Design review of the part built by this model. Coordinates are the model's own, in mm. A direction names the side the tool comes from. Round coordinates to 2 decimals unless told otherwise and drop trailing zeros. Loops run counter-clockwise (first coordinate to the right, second up) from the corner with the lowest first, then second, coordinate; pieces in that order, holes last. Notation, with made-up numbers: (36.25, 66) -> (42.25, 66) arc R20 ccw to (42.25, 92) -> close; hole circle Ø7 at (25, -31). An arc over 180 degrees is marked (long way). Answer as CSV lines item,"result". Start each with the question number.
```python
from build123d import *

# Parameters (mm, degrees)
LOFT1_DEPTH = 254
LOFT1_DRAFT = -8.0697267
SHELL1_T    = -19.05


# Read off the part's stored shape, not the designer's step: Loft1
with BuildPart() as part:
    # Loft1 outline → Loft1 (with draft: the straight prism first)
    with BuildSketch(Plane(origin=(0, -254, 0), x_dir=(1, 0, 0), z_dir=(0, 1, 0))):
        Polygon((45.71024071, -79.172459336), (70.032151779, -58.763952728), (85.907151779, -31.267646158), (91.42048142, 0), (85.907151779, 31.267646158), (70.032151779, 58.763952728), (45.71024071, 79.172459336), (15.875, 90.031598886), (-15.875, 90.031598886), (-45.71024071, 79.172459336), (-70.032151779, 58.763952728), (-85.907151779, 31.267646158), (-91.42048142, 0), (-85.907151779, -31.267646158), (-70.032151779, -58.763952728), (-45.71024071, -79.172459336), (-15.875, -90.031598886), (15.875, -90.031598886), align=None)
    extrude(amount=LOFT1_DEPTH)
    # Loft1: the draft: its side faces are tilted about the plane it starts from
    loft1_sides = [part.faces().sort_by_distance(p)[0] for p in [
        (57.871196245, -127, 68.968206032),
        (77.969651779, -127, 45.015799443),
        (88.6638166, -127, 15.633823079),
        (88.663816599, -127, -15.633823079),
        (77.969651779, -127, -45.015799443),
        (57.871196244, -127, -68.968206032),
        (30.792620355, -127, -84.602029111),
        (0, -127, -90.031598886),
        (-30.792620355, -127, -84.602029111),
        (-57.871196245, -127, -68.968206032),
        (-77.969651779, -127, -45.015799443),
        (-88.6638166, -127, -15.633823079),
        (-88.663816599, -127, 15.633823079),
        (-77.969651779, -127, 45.015799443),
        (-57.871196244, -127, 68.968206032),
        (-30.792620355, -127, 84.602029111),
        (0, -127, 90.031598886),
        (30.792620355, -127, 84.602029111),
    ]]
    draft(loft1_sides, Plane(origin=(0, -254, 0), x_dir=(1, 0, 0), z_dir=(0, 1, 0)), LOFT1_DRAFT)

    # Shell1
    shell1_openings = [part.faces().sort_by_distance(p)[0] for p in [
        (0, 0, 0),
        (0, -254, 0),
    ]]
    offset(amount=SHELL1_T, openings=shell1_openings, kind=Kind.INTERSECTION)


solid = part.part
```
Q1. Add section B-B, the plane z = -13.5. Give the boundary of the cut face in (x, y), and give its area (3 significant figures).
Q2. For pin 1 Ø3 at (y, z) = (-101.5, -60) entering from +X; pin 2 Ø8 at (y, z) = (-192, 62) entering from -X; pin 3 Ø2 at (x, y) = (-18, -45.5) entering from -Z, all flat-tipped, find the tip position at first contact; note any pin that passes through.
Q3. To check wall thickness, follow probe 1 along Z at (x, y) = (14, -168.5); probe 2 along X at (y, z) = (-204, 26); probe 3 along X at (y, z) = (-136, 50). State the ranges of each line that lie inside material, in increasing order. Write a range as from..to.
Q4. Mouldability with a two-part tool opening along Y and no side actions: class faces 3 (the flat face through (-76.814, -128.778, 44.044)), 4 (the flat face through (93.19, -128.78, 54.16)) as pulls with the +Y half, pulls with the -Y half, needs draft (parallel to the pull), parting line crosses it, or undercut.
Q5. Add section C-C, the plane z = 98.5. Give the boundary of the cut face in (x, y).
Q6. Add section A-A, the plane x = 6. Give the boundary of the cut face in (y, z).
Q7. Machinability: for faces 1 (the flat face through (93.501, -128.778, -53.623)), 2 (the flat face through (87.154, -128.778, 15.635)), which of the approach directions +Z, -Z, +X, -X, +Y, -Y give a long, thin tool a straight path to every point of the face, cutting with its end or side? Answer none if there is none.
Worked answers:
1,outline,"(-125.61, 0) -> (-89.04, -254) -> (-69.5, -254) -> (-106.07, 0) -> close; (69.5, -254) -> (89.04, -254) -> (125.61, 0) -> (106.07, 0) -> close"
1,area,"9,920 mm^2"
2,pin 1,"stops at x = 95.19"
2,pin 2,"stops at x = -80.71"
2,pin 3,"stops at z = -119.73"
3,probe 1,"z = -102.15..-82.91, 82.91..102.15"
3,probe 2,"x = -94.03..-74.5, 74.5..94.03"
3,probe 3,"x = -94.41..-72.19, 72.19..94.41"
4,face 3,"pulls with the +Y half"
4,face 4,"pulls with the -Y half"
5,outline,"(-78.7, 0) -> (-56.87, -98.98) -> (-17.37, -194.27) -> (17.37, -194.27) -> (56.87, -98.98) -> (78.7, 0) -> (41.65, 0) -> (17.37, -58.57) -> (-17.37, -58.57) -> (-41.65, 0) -> close"
6,outline,"(-254, -90.03) -> (0, -126.04) -> (0, -106.8) -> (-254, -70.79) -> close; (-254, 70.79) -> (0, 106.8) -> (0, 126.04) -> (-254, 90.03) -> close"
7,face 1,"-Z, +X, -Y"
7,face 2,"+Y"
